Check sheet for the modelled part. Datum: model origin and axes. Units: mm. Face numbers are marked on the shaded views. A direction names the side the tool comes from. Round coordinates to 2 decimals unless told otherwise and drop trailing zeros. Write each loop counter-clockwise with the first axis right and the second up, starting at its lowest first coordinate (ties: lowest second). Pieces come first, ordered by that corner, then holes. Notation, with made-up numbers: (-2.5, 64) -> (49.5, 64) arc R23 ccw to (49.5, 79) -> close; hole circle Ø4 at (50.25, 30.25). An arc over 180 degrees is marked (long way). One line per item, written item: value.
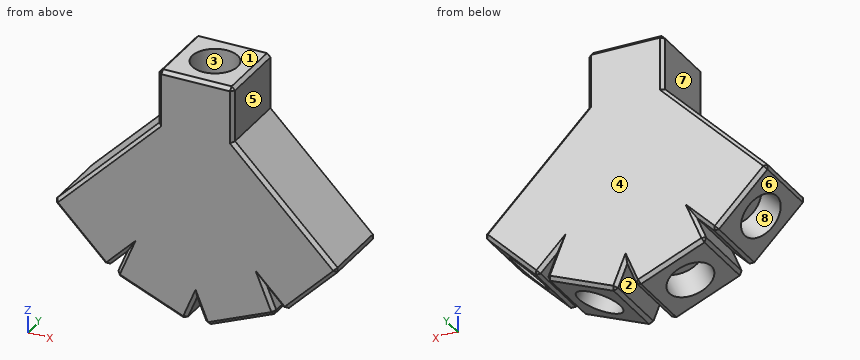
from build123d import *

# Parameters (mm, degrees)
BOSS_EXTRUDE1_DEPTH = 11
SKETCH5_R           = 1.25
CUT_EXTRUDE3_DEPTH  = 21
SKETCH6_R           = 1.25
CUT_EXTRUDE4_DEPTH  = 14
SKETCH7_R           = 1.25
CUT_EXTRUDE5_DEPTH  = 14
SKETCH8_R           = 1.25
CUT_EXTRUDE6_DEPTH  = 21
SKETCH9_W           = 11
SKETCH9_H           = 11
BOSS_EXTRUDE2_DEPTH = 8
SKETCH10_R          = 1.25
CUT_EXTRUDE7_DEPTH  = 18
SKETCH12_R          = 3.302
CUT_EXTRUDE9_DEPTH  = 4
SKETCH18_W          = 11
SKETCH18_H          = 11
SKETCH18_R          = 3.302
BOSS_EXTRUDE3_DEPTH = 4
SKETCH19_W          = 11
SKETCH19_H          = 11
SKETCH19_R          = 3.302
BOSS_EXTRUDE4_DEPTH = 4
SKETCH20_W          = 11
SKETCH20_H          = 11
SKETCH20_R          = 3.302
BOSS_EXTRUDE5_DEPTH = 4
SKETCH22_W          = 11
SKETCH22_H          = 11
SKETCH22_R          = 3.302
BOSS_EXTRUDE7_DEPTH = 4
CHAMFER1_SIZE       = 0.5


with BuildPart() as part:
    # Sketch2 → Boss-Extrude1 (new body)
    with BuildSketch(Plane(origin=(0, 0, 0), x_dir=(1, 0, 0), z_dir=(0, 1, 0))):
        Polygon((0, 24.4285418), (-10.162674858, 20.219024044), (-17.940849451, 12.440849451), (-5.5, 0), (5.5, 0), (17.940849451, 12.440849451), (10.162674858, 20.219024044), align=None)
    extrude(amount=BOSS_EXTRUDE1_DEPTH)

    # Sketch5 → Cut-Extrude3 (cut)
    with BuildSketch(Plane(origin=(15.190849451, 0, -15.190849451), x_dir=(-0.707106781, 0, -0.707106781), z_dir=(0.707106781, 0, -0.707106781))):
        with Locations((1.610912703, 5.5)):
            Circle(SKETCH5_R)
    extrude(amount=-CUT_EXTRUDE3_DEPTH, mode=Mode.SUBTRACT)

    # Sketch6 → Cut-Extrude4 (cut)
    with BuildSketch(Plane(origin=(8.636793781, 0, -20.85106468), x_dir=(-0.923879533, 0, -0.382683432), z_dir=(0.382683432, 0, -0.923879533))):
        with Locations((3.848398224, 5.5)):
            Circle(SKETCH6_R)
    extrude(amount=-CUT_EXTRUDE4_DEPTH, mode=Mode.SUBTRACT)

    # Sketch7 → Cut-Extrude5 (cut)
    with BuildSketch(Plane(origin=(-8.636793781, 0, -20.85106468), x_dir=(-0.923879533, 0, 0.382683432), z_dir=(-0.382683432, 0, -0.923879533))):
        with Locations((-3.848398224, 5.5)):
            Circle(SKETCH7_R)
    extrude(amount=-CUT_EXTRUDE5_DEPTH, mode=Mode.SUBTRACT)

    # Sketch8 → Cut-Extrude6 (cut)
    with BuildSketch(Plane(origin=(-15.190849451, 0, -15.190849451), x_dir=(-0.707106781, 0, 0.707106781), z_dir=(-0.707106781, 0, -0.707106781))):
        with Locations((-1.610912703, 5.5)):
            Circle(SKETCH8_R)
    extrude(amount=-CUT_EXTRUDE6_DEPTH, mode=Mode.SUBTRACT)

    # Sketch9 → Boss-Extrude2 (add)
    with BuildSketch(Plane.XY):
        with Locations((0, 5.5)):
            Rectangle(SKETCH9_W, SKETCH9_H)
    extrude(amount=BOSS_EXTRUDE2_DEPTH)

    # Sketch10 → Cut-Extrude7 (cut)
    with BuildSketch(Plane.XY.offset(8)):
        with Locations((0, 5.5)):
            Circle(SKETCH10_R)
    extrude(amount=-CUT_EXTRUDE7_DEPTH, mode=Mode.SUBTRACT)

    # Sketch12 → Cut-Extrude9 (cut)
    with BuildSketch(Plane.XY.offset(8)):
        with Locations((0, 5.5)):
            Circle(SKETCH12_R)
    extrude(amount=-CUT_EXTRUDE9_DEPTH, mode=Mode.SUBTRACT)

    # Sketch18 → Boss-Extrude3 (add)
    with BuildSketch(Plane(origin=(15.190849451, 0, -15.190849451), x_dir=(-0.707106781, 0, -0.707106781), z_dir=(0.707106781, 0, -0.707106781))):
        with Locations((1.610912703, 5.5)):
            Rectangle(SKETCH18_W, SKETCH18_H)
        with Locations((1.610912703, 5.5)):
            Circle(SKETCH18_R, mode=Mode.SUBTRACT)
    extrude(amount=BOSS_EXTRUDE3_DEPTH)

    # Sketch19 → Boss-Extrude4 (add)
    with BuildSketch(Plane(origin=(8.636793781, 0, -20.85106468), x_dir=(-0.923879533, 0, -0.382683432), z_dir=(0.382683432, 0, -0.923879533))):
        with Locations((3.848398224, 5.5)):
            Rectangle(SKETCH19_W, SKETCH19_H)
        with Locations((3.848398224, 5.5)):
            Circle(SKETCH19_R, mode=Mode.SUBTRACT)
    extrude(amount=BOSS_EXTRUDE4_DEPTH)

    # Sketch20 → Boss-Extrude5 (add)
    with BuildSketch(Plane(origin=(-8.636793781, 0, -20.85106468), x_dir=(-0.923879533, 0, 0.382683432), z_dir=(-0.382683432, 0, -0.923879533))):
        with Locations((-3.848398224, 5.5)):
            Rectangle(SKETCH20_W, SKETCH20_H)
        with Locations((-3.848398224, 5.5)):
            Circle(SKETCH20_R, mode=Mode.SUBTRACT)
    extrude(amount=BOSS_EXTRUDE5_DEPTH)

    # Sketch22 → Boss-Extrude7 (add)
    with BuildSketch(Plane(origin=(-15.190849451, 0, -15.190849451), x_dir=(-0.707106781, 0, 0.707106781), z_dir=(-0.707106781, 0, -0.707106781))):
        with Locations((-1.610912703, 5.5)):
            Rectangle(SKETCH22_W, SKETCH22_H)
        with Locations((-1.610912703, 5.5)):
            Circle(SKETCH22_R, mode=Mode.SUBTRACT)
    extrude(amount=BOSS_EXTRUDE7_DEPTH)

    # Chamfer1
    chamfer1_edges = [part.edges().sort_by_distance(p)[0] for p in [
        (16.880189279, 0, -19.158363872),
        (20.769276575, 5.5, -15.269276575),
        (12.991101982, 5.5, -23.047451168),
        (11.57688842, 0, -21.633237606),
        (16.880189279, 11, -19.158363872),
        (11.57688842, 11, -21.633237606),
        (11.693408587, 5.5, -23.914542174),
        (6.612071158, 0, -26.019301052),
        (1.530733729, 5.5, -28.12405993),
        (6.612071158, 11, -26.019301052),
        (10.928041722, 11, -22.066783109),
        (10.928041722, 0, -22.066783109),
        (0.765366865, 0, -26.276300865),
        (0.765366865, 11, -26.276300865),
        (-1.530733729, 5.5, -28.12405993),
        (-6.612071158, 0, -26.019301052),
        (-11.693408587, 5.5, -23.914542174),
        (-6.612071158, 11, -26.019301052),
        (-0.765366865, 11, -26.276300865),
        (-0.765366865, 0, -26.276300865),
        (-10.928041722, 0, -22.066783109),
        (-10.928041722, 11, -22.066783109),
        (-13.134638288, 11, -7.634638288),
        (-12.991101982, 5.5, -23.047451168),
        (-16.880189279, 0, -19.158363872),
        (-20.769276575, 5.5, -15.269276575),
        (-16.880189279, 11, -19.158363872),
        (-11.57688842, 11, -21.633237606),
        (-11.57688842, 0, -21.633237606),
        (13.134638288, 11, -7.634638288),
        (-5.5, 11, 4),
        (-5.5, 0, 4),
        (5.5, 0, 4),
        (5.5, 11, 4),
        (-5.5, 5.5, 8),
        (0, 0, 8),
        (5.5, 5.5, 8),
        (13.134638288, 0, -7.634638288),
        (0, 11, 8),
        (-13.134638288, 0, -7.634638288),
    ]]
    chamfer(chamfer1_edges, length=CHAMFER1_SIZE)


solid = part.part
Item 1: Tool access check on the marked faces 1, 2, 3, 4 and 5. Record the directions out of +Z, -Z, +X, -X, +Y, -Y that give a thin tool (end or side, any length) a straight path to the whole face; none if there is none.
Answer:
face 1: +Z, +X, -X, +Y, -Y
face 2: -Z, +Y, -Y
face 3: +Z
face 4: +Z, -Z, +X, -X, +Y
face 5: +Z, +X, +Y, -Y
Item 2: Sectioned sample at A-A on z = 1.5. Enter the section's corners in (x, y), and give its area (3 significant figures).
Answer:
outline: (-5.5, 0.5) -> (-5, 0) -> (5, 0) -> (5.5, 0.5) -> (5.5, 10.5) -> (5, 11) -> (-5, 11) -> (-5.5, 10.5) -> close; hole circle Ø2.5 at (0, 5.5)
area: 116 mm^2
Item 3: Thickness scan on line 1 (Y direction, x = 0, z = -4.5); line 2 (Y direction, x = 0, z = 6.75); line 3 (X direction, y = 7.75, z = -22). Record the ranges inside material, lowest first.
Answer:
line 1: y = 0 to 4.25, 6.75 to 11
line 2: y = 0 to 2.2, 8.8 to 11
line 3: x = -14.04 to -11.94, -10.9 to -7.56, -5.86 to 5.86, 7.56 to 10.9, 11.94 to 14.04
Item 4: Sectioned sample at C-C on y = 5.5. Count the separate pieces of the cut face and the enclosed holes in it, and give its area (3 significant figures).
Answer:
separate pieces: 5
enclosed holes: 0
area: 496 mm^2
Item 5: Depth check by flat-ended pin: P1, Ø2, axis at y = 3.5, z = 5, coming from the +X side; P2, Ø6, axis at y = 5, z = 5, coming from the -X side; P3, Ø5, axis at y = 8, z = -1.5, coming from the -X side. Enter the tip coordinate at first touch or a pass-through.
Answer:
P1: stops at x = 5.5
P2: stops at x = -5.5
P3: stops at x = -9.5
Item 6: Sectioned sample at B-B on y = 9.25. Enter the section's corners in (x, z).
Answer:
outline: (-20.42, -15.62) -> (-13.34, -22.69) -> (-12.64, -22.69) -> (-10.16, -20.22) -> (-11.5, -23.45) -> (-11.23, -24.11) -> (-1.99, -27.93) -> (-1.34, -27.66) -> (0, -24.43) -> (1.34, -27.66) -> (1.99, -27.93) -> (11.23, -24.11) -> (11.5, -23.45) -> (10.16, -20.22) -> (12.64, -22.69) -> (13.34, -22.69) -> (20.42, -15.62) -> (20.42, -14.92) -> (5.5, 0) -> (5.5, 7.5) -> (5, 8) -> (-5, 8) -> (-5.5, 7.5) -> (-5.5, 0) -> (-20.42, -14.92) -> close
Item 7: Mould release check, pull along Z, two halves, no side actions. Record for the marked faces 6, 7 and 8: pulls with the +Z half, pulls with the -Z half, needs draft (parallel to the pull), parting line crosses it, or undercut.
Answer:
face 6: pulls with the -Z half
face 7: needs draft
face 8: undercut
